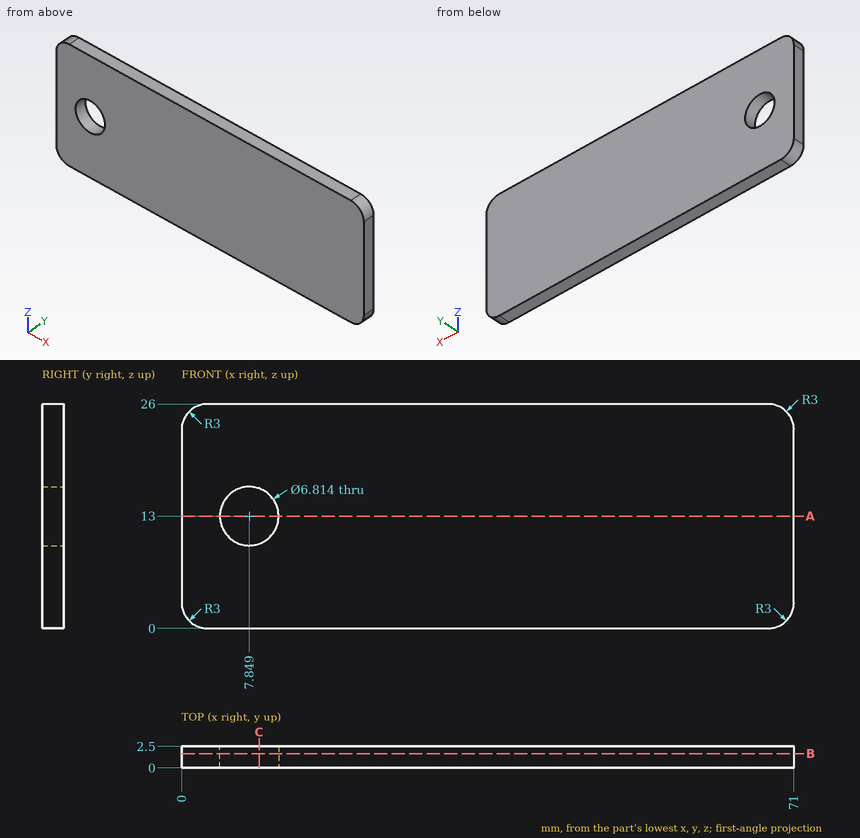
Input: dimensioned drawing with shaded views. Units: mm. Origin: part minimum x, y, z. Give positions to 0.01 mm unless a question says otherwise; leave off trailing zeros. Write each loop counter-clockwise with the first axis right and the second up, starting at its lowest first coordinate (ties: lowest second). Pieces come first, ordered by that corner, then holes. Notation, with made-up numbers: M 67.25,57 L 98.25,57 A22 cw 98.25,77 Z; hole C 70,38 d3. An arc over 180 degrees is marked long. Return JSON: item names as keys, results as strings. Group by question number.
1) Material intervals for line 1 along Z through (x, y) = (5, 2.1); line 2 along Z through (x, y) = (10, 1.2); line 3 along X through (y, z) = (1.5, 24.25), sorted ascending. Write a range as [from, to].
2) Cut plane C-C, the plane x = 9. Output: boundary loops of the cut face in (y, z).
3) Cut plane A-A, the plane z = 13. Output: boundary loops of the cut face in (x, y) (1 decimal).
4) Cut plane B-B, the plane y = 1.65. Output: boundary loops of the cut face in (x, z) (1 decimal).
5) Pin query (flat end, axial travel): P1, Ø4, axis at x = 24, z = 19.5, coming from the -Y side. Return the tip coordinate at first contact, or that it passes through.
Recorded:
{
 "1": {"line 1": "z = [0, 11.13], [14.87, 26]", "line 2": "z = [0, 10.36], [15.64, 26]", "line 3": "x = [0.27, 70.73]"},
 "2": {"outline": "M 0,0 L 2.5,0 L 2.5,9.79 L 0,9.79 Z; M 0,16.21 L 2.5,16.21 L 2.5,26 L 0,26 Z"},
 "3": {"outline": "M 0,0 L 4.4,0 L 4.4,2.5 L 0,2.5 Z; M 11.3,0 L 71,0 L 71,2.5 L 11.3,2.5 Z"},
 "4": {"outline": "M 0,3 A3 ccw 3,0 L 68,0 A3 ccw 71,3 L 71,23 A3 ccw 68,26 L 3,26 A3 ccw 0,23 Z; hole C 7.8,13 d6.8"},
 "5": {"P1": "stops at y = 0"}
}
